Geometry: final body of the model. Coordinates: model frame, mm. Face numbers are marked on the shaded views. A direction names the side the tool comes from. Round coordinates to 2 decimals unless told otherwise and drop trailing zeros. Write each loop counter-clockwise with the first axis right and the second up, starting at its lowest first coordinate (ties: lowest second). Pieces come first, ordered by that corner, then holes.
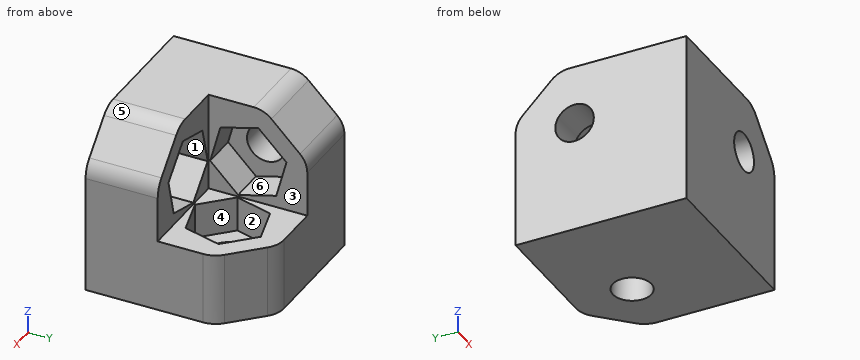
from build123d import *

# Parameters (mm, degrees)
IZIM1_W                     = 15
IZIM1_H                     = 15
IZIM1_R                     = 1.55
Y_KSEKLIK_EKSTR_ZYON1_DEPTH = 3
Y_KSEKLIK_EKSTR_ZYON2_DEPTH = 12
IZIM3_R                     = 1.55
KES_EKSTR_ZYON1_DEPTH       = 4
IZIM4_R                     = 1.55
KES_EKSTR_ZYON2_DEPTH       = 4
Y_KSEKLIK_EKSTR_ZYON3_DEPTH = 2.8
Y_KSEKLIK_EKSTR_ZYON4_DEPTH = 2.8
Y_KSEKLIK_EKSTR_ZYON5_DEPTH = 2.8
KES_EKSTR_ZYON3_DEPTH       = 3
KES_EKSTR_ZYON4_DEPTH       = 3
KES_EKSTR_ZYON5_DEPTH       = 3
IZIM13_W                    = 2.049280952
IZIM13_H                    = 12.849743754
KES_EKSTR_ZYON6_DEPTH       = 16
IZIM14_W                    = 1.259740945
IZIM14_H                    = 10.270148586
KES_EKSTR_ZYON7_DEPTH       = 16
IZIM15_W                    = 10.270148586
IZIM15_H                    = 1.259740945
KES_EKSTR_ZYON8_DEPTH       = 16
RADYUS1_R                   = 2


with BuildPart() as part:
    # Çizim1 → Yükseklik-Ekstrüzyon1 (new body)
    with BuildSketch(Plane.XY):
        with Locations((7.5, -7.5)):
            Rectangle(IZIM1_W, IZIM1_H)
        with Locations((9, -6)):
            Circle(IZIM1_R, mode=Mode.SUBTRACT)
    extrude(amount=Y_KSEKLIK_EKSTR_ZYON1_DEPTH)

    # Çizim2 → Yükseklik-Ekstrüzyon2 (add)
    with BuildSketch(Plane.XY.offset(3)):
        Polygon((0, 0), (0, -15), (15, -15), (15, -12), (3, -12), (3, 0), align=None)
    extrude(amount=Y_KSEKLIK_EKSTR_ZYON2_DEPTH)

    # Çizim3 → Kes-Ekstrüzyon1 (cut, through all)
    with BuildSketch(Plane(origin=(0, -12, 0), x_dir=(1, 0, 0), z_dir=(0, 1, 0))):
        with Locations((9, -9)):
            Circle(IZIM3_R)
    extrude(amount=-KES_EKSTR_ZYON1_DEPTH, mode=Mode.SUBTRACT)

    # Çizim4 → Kes-Ekstrüzyon2 (cut, through all)
    with BuildSketch(Plane(origin=(3, 0, 0), x_dir=(0, 0, -1), z_dir=(1, 0, 0))):
        with Locations((-9, -6)):
            Circle(IZIM4_R)
    extrude(amount=-KES_EKSTR_ZYON2_DEPTH, mode=Mode.SUBTRACT)

    # Çizim5 → Yükseklik-Ekstrüzyon3 (add)
    with BuildSketch(Plane.XY.offset(3)):
        Polygon((13.740259055, -4.729851414), (10.270148586, -1.259740945), (3, -1.259740945), (3, -12), (13.740259055, -12), align=None)
        Polygon((12.067226447, -5.178139151), (9.821860849, -2.932773553), (6.754634402, -3.754634402), (5.932773553, -6.821860849), (8.178139151, -9.067226447), (11.245365598, -8.245365598), align=None, mode=Mode.SUBTRACT)
    extrude(amount=Y_KSEKLIK_EKSTR_ZYON3_DEPTH)

    # Çizim6 → Yükseklik-Ekstrüzyon4 (add)
    with BuildSketch(Plane(origin=(0, -12, 0), x_dir=(1, 0, 0), z_dir=(0, 1, 0))):
        Polygon((10.270148586, -13.740259055), (13.740259055, -10.270148586), (13.740259055, -3), (3, -3), (3, -13.740259055), (5.529889531, -13.740259055), align=None)
        Polygon((12.067226447, -9.821860849), (11.245365598, -6.754634402), (8.178139151, -5.932773553), (5.932773553, -8.178139151), (6.754634402, -11.245365598), (9.821860849, -12.067226447), align=None, mode=Mode.SUBTRACT)
    extrude(amount=Y_KSEKLIK_EKSTR_ZYON4_DEPTH)

    # Çizim7 → Yükseklik-Ekstrüzyon5 (add)
    with BuildSketch(Plane(origin=(3, 0, 0), x_dir=(0, 0, -1), z_dir=(1, 0, 0))):
        Polygon((-10.270148586, -1.259740945), (-13.740259055, -4.729851414), (-13.740259055, -12), (-3, -12), (-3, -1.259740945), align=None)
        Polygon((-11.245365598, -8.245365598), (-8.178139151, -9.067226447), (-5.932773553, -6.821860849), (-6.754634402, -3.754634402), (-9.821860849, -2.932773553), (-12.067226447, -5.178139151), align=None, mode=Mode.SUBTRACT)
    extrude(amount=Y_KSEKLIK_EKSTR_ZYON5_DEPTH)

    # Çizim9 → Kes-Ekstrüzyon3 (cut)
    with BuildSketch(Plane.XY.offset(3)):
        Polygon((9.01040764, 0), (15, -5.98959236), (15, 0), align=None)
    extrude(amount=-KES_EKSTR_ZYON3_DEPTH, mode=Mode.SUBTRACT)

    # Çizim10 → Kes-Ekstrüzyon4 (cut)
    with BuildSketch(Plane(origin=(0, -12, 0), x_dir=(1, 0, 0), z_dir=(0, 1, 0))):
        Polygon((15, -9.01040764), (9.01040764, -15), (15, -15), align=None)
    extrude(amount=-KES_EKSTR_ZYON4_DEPTH, mode=Mode.SUBTRACT)

    # Çizim11 → Kes-Ekstrüzyon5 (cut)
    with BuildSketch(Plane(origin=(3, 0, 0), x_dir=(0, 0, -1), z_dir=(1, 0, 0))):
        Polygon((-9.01040764, 0), (-15, -5.98959236), (-15, 0), align=None)
    extrude(amount=-KES_EKSTR_ZYON5_DEPTH, mode=Mode.SUBTRACT)

    # Çizim13 → Kes-Ekstrüzyon6 (cut)
    with BuildSketch(Plane(origin=(15, 0, 0), x_dir=(0, 0, -1), z_dir=(1, 0, 0))):
        with Locations((-14.764899531, -9.373013496)):
            Rectangle(IZIM13_W, IZIM13_H)
    extrude(amount=-KES_EKSTR_ZYON6_DEPTH, mode=Mode.SUBTRACT)

    # Çizim14 → Kes-Ekstrüzyon7 (cut)
    with BuildSketch(Plane.XY.offset(13.740259055)):
        with Locations((14.370129528, -9.864925707)):
            Rectangle(IZIM14_W, IZIM14_H)
    extrude(amount=-KES_EKSTR_ZYON7_DEPTH, mode=Mode.SUBTRACT)

    # Çizim15 → Kes-Ekstrüzyon8 (cut)
    with BuildSketch(Plane(origin=(13.740259055, 0, 0), x_dir=(0, 0, -1), z_dir=(1, 0, 0))):
        with Locations((-5.135074293, -0.629870473)):
            Rectangle(IZIM15_W, IZIM15_H)
    extrude(amount=-KES_EKSTR_ZYON8_DEPTH, mode=Mode.SUBTRACT)

    # Radyus1
    radyus1_edges = [part.edges().sort_by_distance(p)[0] for p in [
        (2.9, -4.729851414, 13.740259055),
        (2.9, -1.259740945, 10.270148586),
        (13.740259055, -4.729851414, 2.9),
        (10.270148586, -1.259740945, 2.9),
        (13.740259055, -12.1, 10.270148586),
        (10.270148586, -12.1, 13.740259055),
    ]]
    fillet(radyus1_edges, radius=RADYUS1_R)


solid = part.part
1) Section B-B on y = -13.25. Output: boundary loops of the cut face in (x, z), plus the area to 3 significant figures.
2) Draft query along X for the marked faces 4, 5 and 6. Return one class per face: pulls with the +X half, pulls with the -X half, needs draft (parallel to the pull), parting line crosses it, or undercut.
3) Section C-C on z = 9. Output: boundary loops of the cut face in (x, y).
4) Reachability of the marked faces 1, 2 and 3 from +Z, -Z, +X, -X, +Y, -Y: full face, straight path, thin tool, end or side. Return the list, or none.
5) Line query: probe 1 along Z at (x, y) = (9, -14); probe 2 along Y at (x, z) = (9, 1.55). Output: solid intervals per line, ascending.
6) First-contact query: P1, Ø1.8, axis at y = -5.5, z = 8.5, coming from the +X side; P2, Ø2.5, axis at x = 9, z = 9, coming from the -Y side; P3, Ø3, axis at x = 9.5, y = -5.5, coming from the +Z side; P4, Ø6.5, axis at y = -3.5, z = 11, coming from the +X side. Flat tips, straight axial feed; report the tip coordinate or a pass-through.
7) Section D-D on y = -6. Output: boundary loops of the cut face in (x, z).
8) Section A-A on x = 5. Output: boundary loops of the cut face in (y, z), plus the area to 3 significant figures.
Filled in:
1. outline: (0, 0) - (13.74, 0) - (13.74, 9.44) arc R2 ccw to (13.15, 10.86) - (10.86, 13.15) arc R2 ccw to (9.44, 13.74) - (0, 13.74) - close; hole circle Ø3.1 at (9, 9)
1. area: 175 mm2
2. face 4: undercut
2. face 5: pulls with the +X half
2. face 6: needs draft
3. outline: (0, -15) - (7.45, -15) - (7.45, -12) - (6.15, -12) - (6.15, -9.2) - (5.8, -9.2) - (5.8, -8.85) - (3, -8.85) - (3, -7.55) - (0, -7.55) - close; (0, -4.45) - (3, -4.45) - (3, -3.15) - (5.8, -3.15) - (5.8, -1.26) - (0, -1.26) - close; (10.55, -15) - (13.74, -15) - (13.74, -9.2) - (11.85, -9.2) - (11.85, -12) - (10.55, -12) - close
4. face 1: +Y
4. face 2: +Z
4. face 3: +Z, +X, +Y
5. probe 1: z = 0 to 7.45, 10.55 to 13.74
5. probe 2: y = -15 to -7.55, -4.45 to -1.26
6. P1: stops at x = 3
6. P2: passes through
6. P3: stops at z = 3
6. P4: stops at x = 5.8
7. outline: (0, 0) - (7.45, 0) - (7.45, 3) - (6.15, 3) - (6.15, 5.8) - (5.8, 5.8) - (5.8, 6.15) - (3, 6.15) - (3, 7.45) - (0, 7.45) - close; (0, 10.55) - (3, 10.55) - (3, 11.85) - (5.8, 11.85) - (5.8, 13.74) - (0, 13.74) - close; (10.55, 0) - (13.74, 0) - (13.74, 5.8) - (11.85, 5.8) - (11.85, 3) - (10.55, 3) - close
8. outline: (-15, 0) - (-1.26, 0) - (-1.26, 9.44) arc R2 ccw to (-1.85, 10.86) - (-4.14, 13.15) arc R2 ccw to (-5.56, 13.74) - (-15, 13.74) - close; hole (-9.07, 8.18) - (-6.82, 5.93) - (-3.75, 6.75) - (-2.93, 9.82) - (-5.18, 12.07) - (-8.25, 11.25) - close
8. area: 156 mm2
